Work out the finished part from the listing and answer in its coordinate system (mm). A direction names the side the tool comes from. Coordinates: 2 decimals unless noted, no trailing zeros. Loops run counter-clockwise (first coordinate to the right, second up) from the corner with the lowest first, then second, coordinate; pieces in that order, holes last. Notation, with made-up numbers: (-30.5, 57.5) -> (-3.5, 57.5) arc R18 ccw to (-3.5, 82.5) -> close; hole circle Ø5 at (-40, 62). An arc over 180 degrees is marked (long way). Answer as CSV lines item,"result".
```python
from build123d import *

# Parameters (mm, degrees)
SKETCH_1_R      = 6.05
EXTRUDE_1_DEPTH = 5
SKETCH_7_R      = 7
EXTRUDE_6_DEPTH = 1
EXTRUDE_2_DEPTH = 13
EXTRUDE_3_DEPTH = 15


with BuildPart() as part:
    # 草图1 → 凸台-拉伸1 (new body)
    with BuildSketch(Plane.XY):
        Circle(SKETCH_1_R)
    extrude(amount=EXTRUDE_1_DEPTH)

    # 草图7 → 凸台-拉伸6 (add)
    with BuildSketch(Plane.XY.offset(5)):
        Circle(SKETCH_7_R)
    extrude(amount=-EXTRUDE_6_DEPTH)

    # 草图2 → 凸台-拉伸2 (add)
    with BuildSketch(Plane.XY.offset(5)):
        with BuildLine():
            ThreePointArc((4, 0), (1.414213562, 3.741657387), (-3, 2.645751311))
            Line((-3, 2.645751311), (-3, -2.645751311))
            ThreePointArc((-3, -2.645751311), (1.414213562, -3.741657387), (4, 0))
        make_face()
    extrude(amount=EXTRUDE_2_DEPTH)

    # 草图4 → 凸台-拉伸3 (add)
    with BuildSketch(Plane(origin=(0, 0, 0), x_dir=(-1, 0, 0), z_dir=(0, 0, -1))):
        with BuildLine():
            ThreePointArc((4, 0), (-1.645751311, 3.645751311), (-2.645751311, -3))
            Line((-2.645751311, -3), (2.645751311, -3))
            ThreePointArc((2.645751311, -3), (3.645751311, -1.645751311), (4, 0))
        make_face()
    extrude(amount=EXTRUDE_3_DEPTH)


solid = part.part
```
(1) Consider line 1 along Z through (x, y) = (-0.25, -4.25); line 2 along Z through (x, y) = (4.75, 4.75); line 3 along X through (y, z) = (-3.25, 11). Determine where each line is inside the solid, lowest interval first.
Computed values:
line 1,"0 to 5"
line 2,"4 to 5"
line 3,"-2.33 to 2.33"
(2) A cutting plane is placed at A-A, the plane x = 0. Write down the section's boundary in (y, z).
Computed values:
outline,"(-7, 4) -> (-6.05, 4) -> (-6.05, 0) -> (-3, 0) -> (-3, -15) -> (4, -15) -> (4, 0) -> (6.05, 0) -> (6.05, 4) -> (7, 4) -> (7, 5) -> (4, 5) -> (4, 18) -> (-4, 18) -> (-4, 5) -> (-7, 5) -> close"
(3) Which of the six approach directions +Z, -Z, +X, -X, +Y, -Y give full straight-line access (tool end or side, diameter ignored) to faces 1 (the face through (-3.2, 0.1, 5)), 2 (the face through (0, -3, -7)), 3 (the face through (-3, 0, 11)), 4 (the face through (0, -4, 0)), 5 (the face through (0, 1, -15))?
Computed values:
face 1,"+Z"
face 2,"-Z, +X, -X, -Y"
face 3,"+Z, -X, +Y, -Y"
face 4,"-Z"
face 5,"-Z, +X, -X, +Y, -Y"
(4) A cutting plane is placed at C-C, the plane x = -2. Write down the section's boundary in (y, z).
Computed values:
outline,"(-6.71, 4) -> (-5.71, 4) -> (-5.71, 0) -> (-3, 0) -> (-3, -15) -> (3.46, -15) -> (3.46, 0) -> (5.71, 0) -> (5.71, 4) -> (6.71, 4) -> (6.71, 5) -> (3.46, 5) -> (3.46, 18) -> (-3.46, 18) -> (-3.46, 5) -> (-6.71, 5) -> close"
(5) A cutting plane is placed at B-B, the plane z = 1. Write down the section's boundary in (x, y), and give its area (3 significant figures).
Computed values:
outline,"circle Ø12.1 at (0, 0)"
area,"115 mm2"
(6) Flat-ended cylindrical pins translate along their axes: pin 1 Ø4 at (y, z) = (-4, -4) entering from -X; pin 2 Ø2 at (x, z) = (0, -9) entering from -Y; pin 3 Ø3 at (y, z) = (-5, 7.5) entering from -X. Find the tip coordinate at first contact, or state that the pin passes through.
Computed values:
pin 1,"x = -3.46"
pin 2,"y = -3"
pin 3,"x = -1.94"
(7) A cutting plane is placed at D-D, the plane z = -4. Write down the section's boundary in (x, y).
Computed values:
outline,"(-2.65, -3) -> (2.65, -3) arc R4 ccw (long way) to start"
